Check sheet for the drawn part. Datum: minimum x, y, z corner. Units: mm. A direction names the side the tool comes from. Give positions to 0.01 mm unless a question says otherwise; leave off trailing zeros. Loops run counter-clockwise (first coordinate to the right, second up) from the corner with the lowest first, then second, coordinate; pieces in that order, holes last. Notation, with made-up numbers: (-40, 67.25) - (15, 67.25) arc R19 ccw to (15, 104.25) - close; hole circle Ø7 at (-0.75, 25.25). An arc over 180 degrees is marked (long way). Answer in a Markdown table with one row per item.
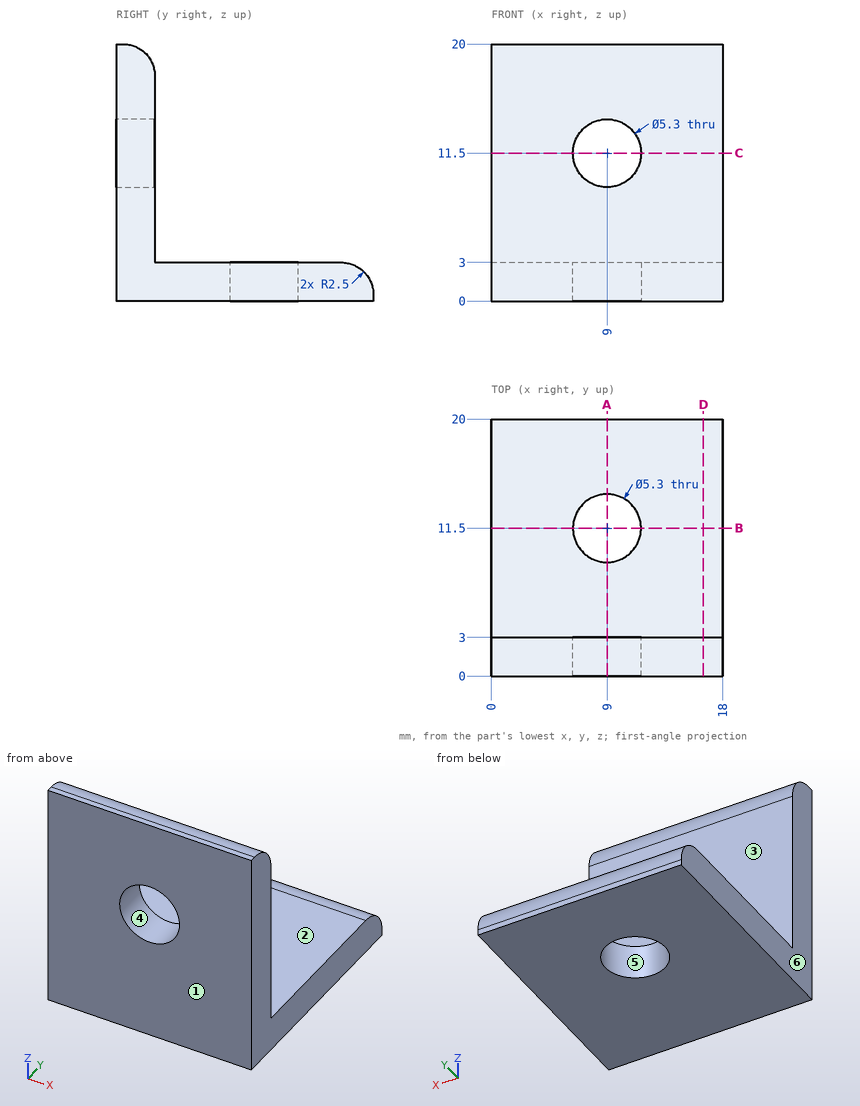
Q1. Draft check along X on the marked faces 3, 4, 5 and 6. Enter one of: +X half, -X half, draft (parallel to the pull), parting line (faces both ways), or undercut.
Completed:
| item | result |
|---|---|
| face 3 | draft |
| face 4 | undercut |
| face 5 | undercut |
| face 6 | -X half |
Q2. Sectioned sample at A-A (x = 9). Record the cut outline in (y, z), and give its area (3 significant figures).
Completed:
| item | result |
|---|---|
| outline | (0, 0) - (8.85, 0) - (8.85, 3) - (3, 3) - (3, 8.85) - (0, 8.85) - close; (0, 14.15) - (3, 14.15) - (3, 17.5) arc R2.5 ccw to (0.5, 20) - (0, 20) - close; (14.15, 0) - (20, 0) - (20, 0.5) arc R2.5 ccw to (17.5, 3) - (14.15, 3) - close |
| area | 76.5 mm^2 |
Q3. Sectioned sample at D-D (x = 16.5). Record the cut outline in (y, z), and give its area (3 significant figures).
Completed:
| item | result |
|---|---|
| outline | (0, 0) - (20, 0) - (20, 0.5) arc R2.5 ccw to (17.5, 3) - (3, 3) - (3, 17.5) arc R2.5 ccw to (0.5, 20) - (0, 20) - close |
| area | 108 mm^2 |
Q4. Sectioned sample at B-B (y = 11.5). Record the cut outline in (x, z).
Completed:
| item | result |
|---|---|
| outline | (0, 0) - (6.35, 0) - (6.35, 3) - (0, 3) - close; (11.65, 0) - (18, 0) - (18, 3) - (11.65, 3) - close |
Q5. Tool access check on the marked faces 1 and 2. Record the directions out of +Z, -Z, +X, -X, +Y, -Y that give a thin tool (end or side, any length) a straight path to the whole face; none if there is none.
Completed:
| item | result |
|---|---|
| face 1 | +Z, -Z, +X, -X, -Y |
| face 2 | +Z, +X, -X, +Y |
Q6. Thickness scan on line 1 (X direction, y = 1.75, z = 11.5); line 2 (Z direction, x = 12.75, y = 17.5). Record the ranges inside material, lowest first.
Completed:
| item | result |
|---|---|
| line 1 | 0 to 6.35, 11.65 to 18 |
| line 2 | 0 to 3 |
Q7. Go/stop test with flat-tipped pins: P1, Ø4.5, axis at x = 9, y = 8, coming from the +Z side; P2, Ø8.5, axis at x = 9, z = 11.5, coming from the +Y side. Record where each tip stops, or that it passes through.
Completed:
| item | result |
|---|---|
| P1 | z = 3 |
| P2 | y = 3 |
